The listing builds one solid part. Answer for the finished solid, in the listing's coordinates (mm). A direction names the side the tool comes from. Give positions to 0.01 mm unless a question says otherwise; leave off trailing zeros. Write each loop counter-clockwise with the first axis right and the second up, starting at its lowest first coordinate (ties: lowest second). Pieces come first, ordered by that corner, then holes. Notation, with made-up numbers: M 52,62 L 71,62 A12 ccw 71,72 Z; hole C 25,-30 d2. An arc over 180 degrees is marked long. Return JSON: item names as keys, results as strings.
from build123d import *

# Parameters (mm, degrees)
SKETCH_2_R      = 4.5
EXTRUDE_1_DEPTH = 7
SKETCH_3_R      = 18
EXTRUDE_2_DEPTH = 13
CHAMFER_1_SIZE  = 1


with BuildPart() as part:
    # 草图2 → 拉伸1 (new body)
    with BuildSketch(Plane(origin=(0, 0, 0), x_dir=(1, 0, 0), z_dir=(0, 1, 0))):
        with BuildLine():
            Line((-12.5, 21.650635095), (-35, 8.660254038))
            ThreePointArc((-35, 8.660254038), (-40, 0), (-35, -8.660254038))
            Line((-35, -8.660254038), (-12.5, -21.650635095))
            ThreePointArc((-12.5, -21.650635095), (0, -25), (12.5, -21.650635095))
            Line((12.5, -21.650635095), (35, -8.660254038))
            ThreePointArc((35, -8.660254038), (40, 0), (35, 8.660254038))
            Line((35, 8.660254038), (12.5, 21.650635095))
            ThreePointArc((12.5, 21.650635095), (0, 25), (-12.5, 21.650635095))
        make_face()
        with Locations(Location((-30, 0, 0), (0, 0, 270))):
            Circle(SKETCH_2_R, mode=Mode.SUBTRACT)
        with Locations(Location((30, 0, 0), (0, 0, 270))):
            Circle(SKETCH_2_R, mode=Mode.SUBTRACT)
    extrude(amount=EXTRUDE_1_DEPTH)

    # 草图3 → 拉伸2 (add)
    with BuildSketch(Plane(origin=(0, 7, 0), x_dir=(1, 0, 0), z_dir=(0, 1, 0))):
        with Locations(Location((0, 0, 0), (0, 0, 90))):
            Circle(SKETCH_3_R)
    extrude(amount=EXTRUDE_2_DEPTH)

    # 草图4 → 切除-旋转2 (revolve, cut)
    with BuildSketch(Plane(origin=(0, 20, 0), x_dir=(1, 0, 0), z_dir=(0, 0, -1)), mode=Mode.PRIVATE) as cut_revolve_2_sk:
        Polygon((0, 20), (11, 20), (11, 4.041451884), (18, 0), (0, 0), align=None)
    revolve(cut_revolve_2_sk.sketch.rotate(Axis((0, -9.575798304, 0), (0, 1, 0)), 90), axis=Axis((0, -9.575798304, 0), (0, 1, 0)), mode=Mode.SUBTRACT)

    # 倒角1
    chamfer_1_edges = [part.edges().sort_by_distance(p)[0] for p in [
        (0, 0, 11),
    ]]
    chamfer(chamfer_1_edges, length=CHAMFER_1_SIZE)


solid = part.part
Item 1: A cutting plane is placed at B-B, the plane z = 0. Write down the section's boundary in (x, y), plus the area to 3 significant figures.
Geometry results:
{"outline": "M -40,0 L -34.5,0 L -34.5,7 L -40,7 Z; M -25.5,0 L -12,0 L -11,1 L -11,15.96 L -18,20 L -18,7 L -25.5,7 Z; M 11,1 L 12,0 L 25.5,0 L 25.5,7 L 18,7 L 18,20 L 11,15.96 Z; M 34.5,0 L 40,0 L 40,7 L 34.5,7 Z", "area": "433 mm2"}
Item 2: Find the intervals of material crossed by line 1 (Z direction, x = -0.5, y = 14); line 2 (Y direction, x = -18, z = 11.5); line 3 (X direction, y = 4, z = -8), in increasing order.
Geometry results:
{"line 1": "z = -17.99 to -10.99, 10.99 to 17.99", "line 2": "y = 0 to 7", "line 3": "x = -36 to -7.55, 7.55 to 36"}
Item 3: Which of the six approach directions +Z, -Z, +X, -X, +Y, -Y give full straight-line access (tool end or side, diameter ignored) to faces 1 (the cylindrical face through (-40, 3, 0)), 2 (the flat face through (-18.3, 7, -0.4))?
Geometry results:
{"face 1": "-X, +Y, -Y", "face 2": "+Y"}
Item 4: Determine the mould class of faces 3 (the flat face through (8, 0, -11)), 4 (the conical face through (11.166, 16.211, 2.48)), 5 (the cylindrical face through (10.74, 8.58, 2.38)), 6 (the flat face through (23.908, 3.451, -15.065)) for opening direction X: +X half, -X half, draft (parallel to the pull), parting line (faces both ways), or undercut.
Geometry results:
{"face 3": "draft", "face 4": "undercut", "face 5": "undercut", "face 6": "+X half"}
Item 5: Given pin 1 Ø3 at (y, z) = (10.5, -12) entering from +X; pin 2 Ø10 at (y, z) = (16.5, -18.5) entering from +X; pin 3 Ø2 at (y, z) = (4.5, -17) entering from +X, each flat-ended and moving along its own axis, determine where each tip first touches the part or whether it passes through.
Geometry results:
{"pin 1": "stops at x = 14.62", "pin 2": "stops at x = 11.91", "pin 3": "stops at x = 22.29"}
Item 6: A cutting plane is placed at D-D, the plane y = 11.75. Write down the section's boundary in (x, z).
Geometry results:
{"outline": "C 0,0 d36; hole C 0,0 d22"}
Item 7: A cutting plane is placed at C-C, the plane y = 3.5. Write down the section's boundary in (x, z).
Geometry results:
{"outline": "M -35,-8.66 L -12.5,-21.65 A25 ccw 12.5,-21.65 L 35,-8.66 A10 ccw 35,8.66 L 12.5,21.65 A25 ccw -12.5,21.65 L -35,8.66 A10 ccw Z; hole C -30,0 d9; hole C 0,0 d22; hole C 30,0 d9"}
Item 8: A cutting plane is placed at A-A, the plane x = 0. Write down the section's boundary in (y, z), plus the area to 3 significant figures.
Geometry results:
{"outline": "M 0,-25 L 7,-25 L 7,-18 L 20,-18 L 15.96,-11 L 1,-11 L 0,-12 Z; M 0,12 L 1,11 L 15.96,11 L 20,18 L 7,18 L 7,25 L 0,25 Z", "area": "349 mm2"}
